```python
from build123d import *

# Parameters (mm, degrees)
SKETCH1_W                    = 12.7
SKETCH1_H                    = 19.525000066
BOSS_EXTRUDE1_DEPTH          = 3
CONVERT_SOLID2_START         = -0.175
CONVERT_SOLID2_OUTLINE_W     = 12.7
CONVERT_SOLID2_OUTLINE_H     = 19.525000066
CONVERT_SOLID2_DEPTH         = 0.175
EDGE_FLANGE1_STRIP_W         = 18.796
EDGE_FLANGE1_STRIP_H         = 3.175
EDGE_FLANGE1_STRIP_CUT_DEPTH = 12.7
EDGE_FLANGE1_DEPTH           = 12.7
M4_CLEARANCE_HOLE4_D         = 4.5
M4_CLEARANCE_HOLE4_DEPTH     = 16.002
M4_CLEARANCE_HOLE4_TIP       = 1.351936393
FILLET1_R                    = 3.175


# Read off the part's stored shape, not the designer's step: Convert-Solid2
# Sheet-metal steps are written as plain solids
with BuildPart() as part:
    # Sketch1 → Boss-Extrude1 (new body)
    with BuildSketch(Plane.XY):
        with Locations((6.35, 9.762500033)):
            Rectangle(SKETCH1_W, SKETCH1_H)
    extrude(amount=BOSS_EXTRUDE1_DEPTH)

    # Convert-Solid2 outline → Convert-Solid2 (add)
    with BuildSketch(Plane.XY.offset(CONVERT_SOLID2_START)):
        with Locations((6.35, 9.762500033)):
            Rectangle(CONVERT_SOLID2_OUTLINE_W, CONVERT_SOLID2_OUTLINE_H)
    extrude(amount=CONVERT_SOLID2_DEPTH)

    # Edge-Flange1 strip (across the edge) → Edge-Flange1 strip cut (cut)
    with BuildSketch(Plane(origin=(0, 0, 3), x_dir=(0, 1, 0), z_dir=(1, 0, 0))):
        with Locations((-3.175, -1.5875)):
            Rectangle(EDGE_FLANGE1_STRIP_W, EDGE_FLANGE1_STRIP_H)
    extrude(amount=EDGE_FLANGE1_STRIP_CUT_DEPTH, mode=Mode.SUBTRACT)

    # Edge-Flange1 section (across the edge) → Edge-Flange1 (add)
    with BuildSketch(Plane(origin=(0, 0, 3), x_dir=(0, 1, 0), z_dir=(1, 0, 0))):
        with BuildLine():
            Line((0, 3.048), (0, 16.350000066))
            Line((0, 16.350000066), (3.175, 16.350000066))
            Line((3.175, 16.350000066), (3.175, 3.048))
            ThreePointArc((3.175, 3.048), (4.067738531, 0.892738531), (6.223, 0))
            Line((6.223, 0), (6.223, -3.175))
            ThreePointArc((6.223, -3.175), (1.822674501, -1.352325499), (0, 3.048))
        make_face()
    extrude(amount=EDGE_FLANGE1_DEPTH)

    # M4 Clearance Hole4
    with Locations(Plane(origin=(0, 3.175, 0), x_dir=(1, 0, 0), z_dir=(0, 1, 0))):
        with Locations((6.35, -12.699000033)):
            Hole(M4_CLEARANCE_HOLE4_D / 2, depth=M4_CLEARANCE_HOLE4_DEPTH)
            with Locations((0, 0, -(M4_CLEARANCE_HOLE4_DEPTH + M4_CLEARANCE_HOLE4_TIP / 2))):  # 118° drill point
                Cone(0, M4_CLEARANCE_HOLE4_D / 2, M4_CLEARANCE_HOLE4_TIP, mode=Mode.SUBTRACT)

    # Fillet1
    fillet1_edges = [part.edges().sort_by_distance(p)[0] for p in [
        (0, 1.5875, 19.350000066),
        (12.7, 1.5875, 19.350000066),
        (0, 19.525000066, 1.4125),
        (12.7, 19.525000066, 1.4125),
    ]]
    fillet(fillet1_edges, radius=FILLET1_R)


solid = part.part
```
CAD build for the part. Positions are in the model's coordinates, mm. A direction names the side the tool comes from. Round coordinates to 2 decimals unless told otherwise and drop trailing zeros. Write each loop counter-clockwise with the first axis right and the second up, starting at its lowest first coordinate (ties: lowest second). Pieces come first, ordered by that corner, then holes. Notation, with made-up numbers: (87.5, 31.25) -> (93.5, 31.25) arc R35 cw to (93.5, 69.25) -> close; hole circle Ø3 at (26.25, 47). An arc over 180 degrees is marked (long way). Answer in a Markdown table with one row per item. Add a question column.
Item 1: Drill centre lines: line 1 (Y direction, x = 9, z = 11.5) (3 decimals); line 2 (Z direction, x = 11.75, y = 9) (3 decimals); line 3 (Z direction, x = 6.35, y = 1.9). Where is each one in solid material? Low to high. Write a range as from..to.
Item 2: Saw through at D-D, the plane x = 3.75. Write the cut outline in (y, z) (3 decimals).
Item 3: Saw through at C-C, the plane y = 2. Write the cut outline in (x, z) (3 decimals), then the cut area to 3 significant figures.
Item 4: Mould opens along Z. For faces 1 (the face through (6.838, 1.565, 14.895)), 2 (the face through (0.905, 18.57, 1.39)), 3 (the face through (6, 13, 3)) say: pulls with the +Z half, pulls with the -Z half, needs draft (parallel to the pull), parting line crosses it, or undercut.
Item 5: Which spindle directions (+Z, -Z, +X, -X, +Y, -Y) get a long thin tool onto all of the face, cutting with end or side? Do faces 4 (the face through (6, 0, 10)), 5 (the face through (6, 3.175, 10)). Say none if no direction does.
Item 6: Saw through at B-B, the plane z = 12. Write the cut outline in (x, y) (3 decimals), then the cut area to 3 significant figures.
Item 7: Saw through at A-A, the plane x = 6.35. Write the cut outline in (y, z) (3 decimals).
Item 8: Drop flat-ended pins along their axis: pin 1 Ø1.5 at (y, z) = (4, 6.5) entering from +X; pin 2 Ø3 at (x, z) = (7.5, 13) entering from +Y (3 decimals); pin 3 Ø6 at (x, y) = (7, 14.5) entering from +Z. Give the stop position or say it passes through.
Findings below:
| question | item | result |
|---|---|---|
| 1 | line 1 | y = 0..3.175 |
| 1 | line 2 | z = -0.175..3 |
| 1 | line 3 | z = 1.57..10.45, 14.95..19.35 |
| 2 | outline | (0, 6.048) arc R6.223 ccw to (6.223, -0.175) -> (19.525, -0.175) -> (19.525, 3) -> (6.223, 3) arc R3.048 cw to (3.175, 6.048) -> (3.175, 19.35) -> (0, 19.35) -> close |
| 3 | outline | (0, 1.477) -> (12.7, 1.477) -> (12.7, 16.175) arc R3.175 ccw to (9.525, 19.35) -> (3.175, 19.35) arc R3.175 ccw to (0, 16.175) -> close; hole circle Ø4.5 at (6.35, 12.699) |
| 3 | area | 207 mm^2 |
| 4 | face 1 | undercut |
| 4 | face 2 | needs draft |
| 4 | face 3 | pulls with the +Z half |
| 5 | face 4 | +Z, -Z, +X, -X, -Y |
| 5 | face 5 | +Z, +X, -X, +Y |
| 6 | outline | (0, 0) -> (4.211, 0) -> (4.211, 3.175) -> (0, 3.175) -> close; (8.489, 0) -> (12.7, 0) -> (12.7, 3.175) -> (8.489, 3.175) -> close |
| 6 | area | 26.7 mm^2 |
| 7 | outline | (0, 6.048) arc R6.223 ccw to (6.223, -0.175) -> (19.525, -0.175) -> (19.525, 3) -> (6.223, 3) arc R3.048 cw to (3.175, 6.048) -> (3.175, 10.449) -> (0, 10.449) -> close; (0, 14.949) -> (3.175, 14.949) -> (3.175, 19.35) -> (0, 19.35) -> close |
| 8 | pin 1 | passes through |
| 8 | pin 2 | stops at y = 3.175 |
| 8 | pin 3 | stops at z = 3 |
